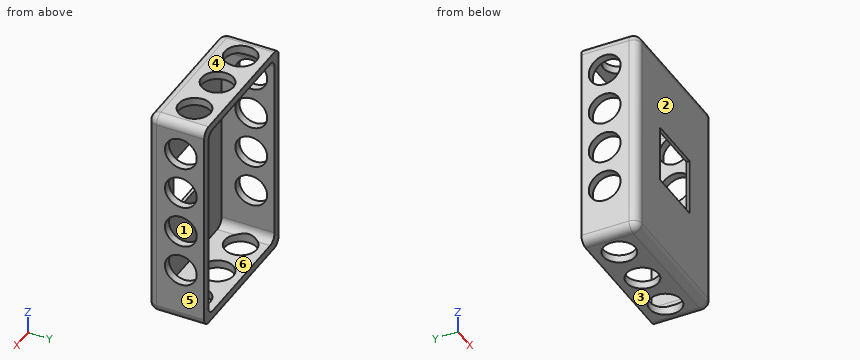
Autodesk Inventor part; units mm, degrees
ref_plane "YZ Plane" through (0, 0, 0) normal (1, 0, 0) x (0, 1, 0)
ref_plane "XZ Plane" through (0, 0, 0) normal (0, 1, 0) x (-1, 0, 0)
ref_plane "XY Plane" through (0, 0, 0) normal (0, 0, 1) x (1, 0, 0)
sketch "Sketch1" plane through (0, 0, 0) normal (0, 1, 0) x (-1, 0, 0)
  line L0 (33.92, 50.615) -> (-33.92, 50.615)
  line L1 (-33.92, 50.615) -> (-33.92, -50.615)
  line L2 (-33.92, -50.615) -> (33.92, -50.615)
  line L3 (33.92, -50.615) -> (33.92, 50.615)
  line L4 (33.92, 50.615) -> (-33.92, -50.615) construction
  line L5 (-33.92, 50.615) -> (33.92, -50.615) construction
  point P0 (0, 0)
  dimension "d0" = 67.84
  dimension "d1" = 101.23
extrude "Extrusion1" add sketch "Sketch1" along normal blind 26.5
fillet "Fillet1" radius 4 8 edges at (33.92, 13.25, 50.615) (33.92, 0, 0) (33.92, 13.25, -50.615) (-33.92, 13.25, -50.615) (0, 0, -50.615) (0, 0, 50.615) (-33.92, 13.25, 50.615) (-33.92, 0, 0)
sketch "Sketch2" plane through (0, 26.5, 0) normal (0, 1, 0) x (1, 0, 0)
  line L0 (30.2, 46.895) -> (-30.2, 46.895)
  line L1 (-30.2, 46.895) -> (-30.2, -46.895)
  line L2 (-30.2, -46.895) -> (30.2, -46.895)
  line L3 (30.2, -46.895) -> (30.2, 46.895)
  line L4 (30.2, 46.895) -> (-30.2, -46.895) construction
  line L5 (-30.2, 46.895) -> (30.2, -46.895) construction
  line L6 (-29.92, -50.615) -> (29.92, -50.615)
  line L7 (33.92, -46.615) -> (33.92, 46.615)
  point P0 (0, 0)
  dimension "d5" = 3.72
  dimension "d6" = 3.72
extrude "Extrusion2" cut sketch "Sketch2" against normal blind 25
fillet "Fillet2" radius 4 4 edges at (30.2, 14, -46.895) (30.2, 14, 46.895) (-30.2, 14, -46.895) (-30.2, 14, 46.895)
sketch "Sketch3" plane through (0, 0, 0) normal (0, -1, 0) x (1, 0, 0)
  line L0 (-13.5, -13.5) -> (13.5, -13.5)
  line L1 (13.5, -13.5) -> (13.5, 13.5)
  line L2 (13.5, 13.5) -> (-13.5, 13.5)
  line L3 (-13.5, 13.5) -> (-13.5, -13.5)
  line L4 (-13.5, -13.5) -> (13.5, 13.5) construction
  line L5 (13.5, -13.5) -> (-13.5, 13.5) construction
  point P0 (0, 0)
  dimension "d10" = 27
  dimension "d11" = 27
extrude "Extrusion4" cut sketch "Sketch3" against normal through all
sketch "Sketch4" plane through (-33.92, 4, 46.615) normal (-1, 0, 0) x (0, 0, 1)
  circle A0 centre (-11.226, 11.5) radius 7.5
  circle A1 centre (-31.226, 11.5) radius 7.5
  circle A2 centre (-51.226, 11.5) radius 7.5
  circle A3 centre (-71.226, 11.5) radius 7.5
  line L0 (0, 22.5) -> (0, 0)
  line L1 (-93.23, 22.5) -> (0, 22.5)
  point P0 (-46.615, -4)
  dimension "d17" = 15
  dimension "d18" = 15
  dimension "d19" = 20
  dimension "d20" = 15
  dimension "d21" = 15
  dimension "d22" = 20
  dimension "d23" = 20
  dimension "d24" = 11.226
  dimension "d25" = 11
  dimension "d26" = 11
  dimension "d27" = 11
  dimension "d28" = 11
extrude "Extrusion5" cut sketch "Sketch4" against normal through all
sketch "Sketch5" plane through (29.92, 4, -50.615) normal (0, 0, -1) x (-1, 0, 0)
  line L0 (59.84, 22.5) -> (59.84, 0)
  line L1 (0, 22.5) -> (59.84, 22.5)
  line L2 (59.84, 0) -> (0, 22.5) construction
  line L3 (59.84, 0) -> (0, 0)
  line L4 (59.84, 22.5) -> (0, 0) construction
  circle A0 centre (29.92, 11.25) radius 7.5
  circle A1 centre (50.92, 11.25) radius 7.5
  circle A2 centre (8.92, 11.25) radius 7.5
  line L5 (0, 0) -> (0, 22.5)
  point P0 (29.92, -4)
  dimension "d31" = 15
  dimension "d32" = 15
  dimension "d33" = 15
  dimension "d34" = 21
  dimension "d35" = 21
  dimension "d36" = 8.92
  dimension "d37" = 8.92
extrude "Extrusion6" cut sketch "Sketch5" against normal through all contours A0 | A1 | A2
properties part number "TopCover" material "ABS Plastic"
Work out the finished part from the listing and answer in its coordinate system (mm). Face numbers are marked on the shaded views. A direction names the side the tool comes from. Round coordinates to 2 decimals unless told otherwise and drop trailing zeros. Order: outer loops, then holes, each group sorted by start corner. A loop starts at its lowest first (then second) coordinate and runs counter-clockwise, first axis right, second up. Notation, with made-up numbers: M 63,41.25 L 101,41.25 A15 cw 101,61.25 Z; hole C -30.5,44 d3. An arc over 180 degrees is marked long. One line per item, written item: value.
Q1. For the marked faces 1 and 2, determine the directions among +Z, -Z, +X, -X, +Y, -Y from which every point of the face is accessible in a straight line to the end or side of a thin tool.
Derived:
face 1: +Y
face 2: +Z, -Z, +X, -X, -Y
Q2. Find section C-C on y = 24.5. Write down the section's boundary in (x, z) (3 decimals), then the cut area to 3 significant figures.
Derived:
outline: M -33.92,-46.615 A4 ccw -29.92,-50.615 L 29.92,-50.615 A4 ccw 33.92,-46.615 L 33.92,46.615 A4 ccw 29.92,50.615 L -29.92,50.615 A4 ccw -33.92,46.615 Z; hole M -30.2,-42.895 A4 ccw -26.2,-46.895 L 26.2,-46.895 A4 ccw 30.2,-42.895 L 30.2,42.895 A4 ccw 26.2,46.895 L -26.2,46.895 A4 ccw -30.2,42.895 Z
area: 1,200 mm²
Q3. Flat-ended cylindrical pins translate along their axes: pin 1 (8 mm diameter, centred on x = -21.5, z = -0.5, fed in from +Y); pin 2 (1.6 mm diameter, centred on x = 6.5, y = 0.5, fed in from +Z); pin 3 (1.2 mm diameter, centred on y = 1, z = 4.5, fed in from +X). Find the tip coordinate at first contact, or state that the pin passes through.
Derived:
pin 1: y = 1.5
pin 2: z = 49.57
pin 3: x = 33.12
Q4. Find section D-D on z = 14.5. Write down the section's boundary in (x, y).
Derived:
outline: M -33.92,4 A4 ccw -29.92,0 L 29.92,0 A4 ccw 33.92,4 L 33.92,8.05 L 30.2,8.05 L 30.2,1.5 L -30.2,1.5 L -30.2,8.05 L -33.92,8.05 Z; M -33.92,22.95 L -30.2,22.95 L -30.2,26.5 L -33.92,26.5 Z; M 30.2,22.95 L 33.92,22.95 L 33.92,26.5 L 30.2,26.5 Z
Q5. Find section B-B on x = 0. Write down the section's boundary in (y, z) (3 decimals), then the cut area to 3 significant figures.
Derived:
outline: M 0,-46.615 A4 ccw 4,-50.615 L 7.75,-50.615 L 7.75,-46.895 L 1.5,-46.895 L 1.5,-13.5 L 0,-13.5 Z; M 0,13.5 L 1.5,13.5 L 1.5,46.895 L 7.75,46.895 L 7.75,50.615 L 4,50.615 A4 ccw 0,46.615 Z; M 22.75,-50.615 L 26.5,-50.615 L 26.5,-46.895 L 22.75,-46.895 Z; M 22.75,46.895 L 26.5,46.895 L 26.5,50.615 L 22.75,50.615 Z
area: 179 mm²
Q6. Find section A-A on x = 11.5. Write down the section's boundary in (y, z) (3 decimals), then the cut area to 3 significant figures.
Derived:
outline: M 0,-46.615 A4 ccw 4,-50.615 L 26.5,-50.615 L 26.5,-46.895 L 1.5,-46.895 L 1.5,-13.5 L 0,-13.5 Z; M 0,13.5 L 1.5,13.5 L 1.5,46.895 L 26.5,46.895 L 26.5,50.615 L 4,50.615 A4 ccw 0,46.615 Z
area: 290 mm²
Q7. Straight lines are drawn through the part: line 1 (X direction, y = 24.5, z = 1); line 2 (Z direction, x = -0.5, y = 7) (3 decimals); line 3 (X direction, y = 18.75, z = -45). For each, find the intervals that lie inside material, in ascending order.
Derived:
line 1: -33.92 to -30.2, 30.2 to 33.92
line 2: -50.615 to -46.895, 46.895 to 50.615
line 3: -33.92 to -29.6, 29.6 to 33.92
Q8. Determine the mould class of the marked faces 3, 4, 5 and 6 for opening direction Z: released by +Z, released by -Z, zero draft, split by the parting line, or undercut.
Derived:
face 3: released by -Z
face 4: released by +Z
face 5: zero draft
face 6: undercut
